Design review of the part shown in the three views and the two pictorial views. Dimensions are in mm from the part's minimum x, y and z. A direction names the side the tool comes from. Coordinates: 2 decimals unless noted, no trailing zeros. Loops run counter-clockwise (first coordinate to the right, second up) from the corner with the lowest first, then second, coordinate; pieces in that order, holes last. Notation, with made-up numbers: (-40, 9.25) - (-12, 9.25) arc R26 cw to (-12, 40.25) - close; hole circle Ø1 at (-34, 79). An arc over 180 degrees is marked (long way). One line per item, written item: value. Start each with the question number.
1. Take a section at B-B, the plane x = 7.5. State the section outline as (y, z) points, and give its area (3 significant figures).
2. The part is to be moulded in two halves that separate along X. For the marked faces 1, 2 and 3, say which applies: released by +X, released by -X, zero draft, split by the parting line, or undercut.
3. Take a section at A-A, the plane z = 20. State the section outline as (x, y) points.
4. Insertion check: pin 1 (5 mm diameter, centred on y = 6, z = 20.5, fed in from -X); pin 2 (1 mm diameter, centred on y = 9, z = 29, fed in from +X); pin 3 (5 mm diameter, centred on x = 41.5, y = 7, fed in from -Z). Each pin has a flat end and moves straight along its axis. Give the tip position at first contact, or say it passes through.
5. To check wall thickness, follow line 1 (X direction, y = 2.5, z = 2.5); line 2 (Z direction, x = 40, y = 6.25); line 3 (Z direction, x = 69.5, y = 7). State the ranges of each line that lie inside material, in increasing order. Write a range as from..to.
6. For the marked faces 4, 5, 6, 7 and 8, list the 3-axis set-ups (+Z, -Z, +X, -X, +Y, -Y) from which the entire face can be reached by the end or side of a thin tool; tool diameter is ignored.
7. Take a section at D-D, the plane z = 12.5. State the section outline as (x, y) points.
8. Take a section at C-C, the plane y = 5. State the section outline as (x, z) points, and give its area (3 significant figures).
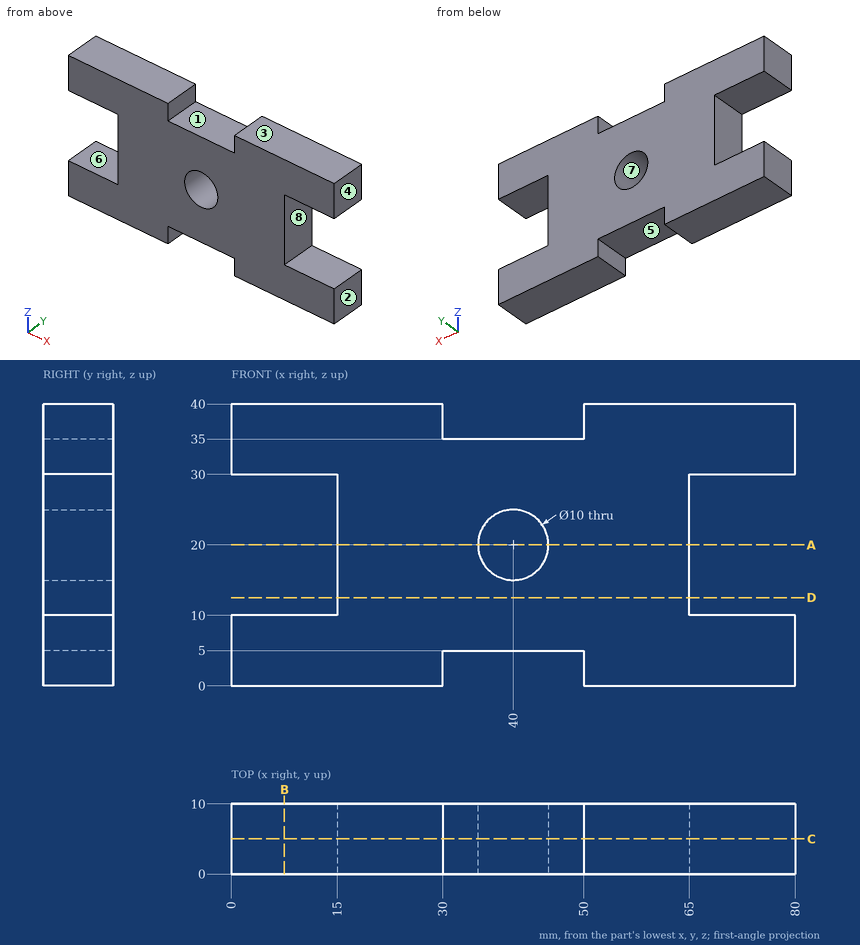
Solutions:
1. outline: (0, 0) - (10, 0) - (10, 10) - (0, 10) - close; (0, 30) - (10, 30) - (10, 40) - (0, 40) - close
1. area: 200 mm2
2. face 1: undercut
2. face 2: released by +X
2. face 3: zero draft
3. outline: (15, 0) - (35, 0) - (35, 10) - (15, 10) - close; (45, 0) - (65, 0) - (65, 10) - (45, 10) - close
4. pin 1: x = 15
4. pin 2: x = 65
4. pin 3: z = 5
5. line 1: 0..30, 50..80
5. line 2: 5..15, 25..35
5. line 3: 0..10, 30..40
6. face 4: +Z, -Z, +X, +Y, -Y
6. face 5: -Z, +Y, -Y
6. face 6: -X, +Y, -Y
6. face 7: +Y, -Y
6. face 8: +X, +Y, -Y
7. outline: (15, 0) - (65, 0) - (65, 10) - (15, 10) - close
8. outline: (0, 0) - (30, 0) - (30, 5) - (50, 5) - (50, 0) - (80, 0) - (80, 10) - (65, 10) - (65, 30) - (80, 30) - (80, 40) - (50, 40) - (50, 35) - (30, 35) - (30, 40) - (0, 40) - (0, 30) - (15, 30) - (15, 10) - (0, 10) - close; hole circle Ø10 at (40, 20)
8. area: 2,320 mm2
